Verification items for the finished model (mm, model axes). Face numbers are marked on the shaded views. Give positions to 0.01 mm unless a question says otherwise; leave off trailing zeros. Order: outer loops, then holes, each group sorted by start corner. A loop starts at its lowest first (then second) coordinate and runs counter-clockwise, first axis right, second up. Notation, with made-up numbers: (14, -22.75) - (73, -22.75) arc R7 ccw to (73, -16.75) - close; hole circle Ø11 at (72.25, 64.5). An arc over 180 degrees is marked (long way). Answer as a JSON object with one key per item and string values.
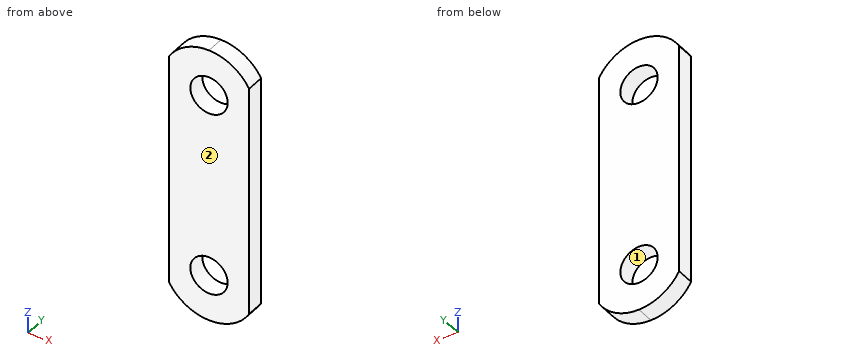
```python
from build123d import *

# Parameters (mm, degrees)
SKETCH1_W               = 10.9728
SKETCH1_H               = 2.4384
EXTRUDE1_DEPTH          = 38.1
F_1_4_20_TAPPED_HOLE1_D = 5.1054
CUT_EXTRUDE1_DEPTH      = 40.723521173


with BuildPart() as part:
    # Sketch1 → Extrude1 (new body)
    with BuildSketch(Plane.XY):
        with Locations((5.4864, 1.2192)):
            Rectangle(SKETCH1_W, SKETCH1_H)
    extrude(amount=EXTRUDE1_DEPTH)

    # 1/4-20 Tapped Hole1 (through all)
    with Locations(Plane(origin=(5.4864, 2.4384, 6.35), x_dir=(0, 0, 1), z_dir=(0, 1, 0))):
        with Locations((0, 0), (25.4, 0)):
            Hole(F_1_4_20_TAPPED_HOLE1_D / 2)

    # Sketch4 → Cut-Extrude1 (cut, through all)
    with BuildSketch(Plane(origin=(0, 2.4384, 0), x_dir=(-1, 0, 0), z_dir=(0, 1, 0))):
        with BuildLine():
            ThreePointArc((0, 3.152827024), (-2.322505912, 0.84434162), (-5.4864, 0))
            Line((-5.4864, 0), (0, 0))
            Line((0, 0), (0, 3.152827024))
        make_face()
        with BuildLine():
            ThreePointArc((-5.4864, 0), (-8.651032451, 0.844765995), (-10.97365738, 3.154298755))
            Line((-10.97365738, 3.154298755), (-10.9728, 0))
            Line((-10.9728, 0), (-5.4864, 0))
        make_face()
        with BuildLine():
            Line((-10.9728, 38.1), (-10.97365738, 34.945701245))
            ThreePointArc((-10.97365738, 34.945701245), (-8.651032451, 37.255234005), (-5.4864, 38.1))
            Line((-5.4864, 38.1), (-10.9728, 38.1))
        make_face()
        with BuildLine():
            Line((0, 38.1), (-5.4864, 38.1))
            ThreePointArc((-5.4864, 38.1), (-2.322505912, 37.25565838), (0, 34.947172976))
            Line((0, 34.947172976), (0, 38.1))
        make_face()
    extrude(amount=-CUT_EXTRUDE1_DEPTH, mode=Mode.SUBTRACT)


solid = part.part
```
(1) Section check A-A (z = 31.75). Record the cut outline in (x, y).
Computed values:
{"outline": "(0, 0) - (2.93, 0) - (2.93, 2.44) - (0, 2.44) - close; (8.04, 0) - (10.97, 0) - (10.97, 2.44) - (8.04, 2.44) - close"}
(2) Material ranges on line 1 along Z through (x, y) = (5.5, 1.65); line 2 along X through (y, z) = (1.6, 31.75); line 3 along Z through (x, y) = (4.75, 1.2), recorded low to high. Write a range as [from, to].
Computed values:
{"line 1": "z = [0, 3.8], [8.9, 29.2], [34.3, 38.1]", "line 2": "x = [0, 2.93], [8.04, 10.97]", "line 3": "z = [0.04, 3.91], [8.79, 29.31], [34.19, 38.06]"}
(3) Gauge pin test, flat end, axial feed: pin 1 Ø4 at (x, z) = (8.5, 30.5) entering from -Y. Record the tip position at first contact, or that the pin passes through.
Computed values:
{"pin 1": "stops at y = 0"}
(4) Release check for a two-part mould opening along X. For the marked faces 1 and 2 record: pulls with the +X half, pulls with the -X half, needs draft (parallel to the pull), parting line crosses it, or undercut.
Computed values:
{"face 1": "undercut", "face 2": "needs draft"}
(5) Section check B-B (y = 0.95). Record the cut outline in (x, z).
Computed values:
{"outline": "(0, 3.15) arc R6.35 ccw to (10.97, 3.15) - (10.97, 34.95) arc R6.35 ccw to (0, 34.95) - close; hole circle Ø5.11 at (5.49, 6.35); hole circle Ø5.11 at (5.49, 31.75)"}
(6) Section check C-C (z = 6.5). Record the cut outline in (x, y).
Computed values:
{"outline": "(0, 0) - (2.94, 0) - (2.94, 2.44) - (0, 2.44) - close; (8.03, 0) - (10.97, 0) - (10.97, 2.44) - (8.03, 2.44) - close"}
